```python
from build123d import *

# Parameters (mm, degrees)
DODANIE_WYCI_GNI_CIE1_DEPTH      = 85
SZKIC2_W                         = 10
SZKIC2_H                         = 10
WYTNIJ_WYCI_GNI_CIE1_DEPTH       = 80
DODANIE_WYCI_GNI_CIE3_DEPTH      = 80
DODANIE_WYCI_GNI_CIE3_DEPTH_BACK = 47
SZKIC4_W                         = 15.782842712
SZKIC4_H                         = 20
DODANIE_WYCI_GNI_CIE4_DEPTH      = 4
SZKIC5_W                         = 4
SZKIC5_H                         = 5
DODANIE_WYCI_GNI_CIE5_DEPTH      = 10
SZKIC6_W                         = 4
SZKIC6_H                         = 5
DODANIE_WYCI_GNI_CIE6_DEPTH      = 10
SFAZOWANIE1_SIZE                 = 1.5


with BuildPart() as part:
    # Szkic1 → Dodanie-wyci_gni_cie1 (new body)
    with BuildSketch(Plane.XY):
        Polygon((7.5, 0), (11.5, 4), (-10.578691808, 4), (-6.578691808, 0), align=None)
    extrude(amount=DODANIE_WYCI_GNI_CIE1_DEPTH)

    # Szkic2 → Wytnij-wyci_gni_cie1 (cut)
    with BuildSketch(Plane.XZ):
        with Locations((0.460654096, 21)):
            Rectangle(SZKIC2_W, SZKIC2_H)
        with Locations((0.460654096, 71)):
            Rectangle(SZKIC2_W, SZKIC2_H)
    extrude(amount=-WYTNIJ_WYCI_GNI_CIE1_DEPTH, mode=Mode.SUBTRACT)



with BuildPart() as body_2:
    # Szkic1_4 → Dodanie-wyci_gni_cie3 (new, two sides: drawn at the far end of the back side and taken through both)
    with BuildSketch(Plane.XY.offset(-DODANIE_WYCI_GNI_CIE3_DEPTH_BACK)):
        Polygon((19.282842712, 4), (23.282842712, 0), (26.717157288, 0), (30.717157288, 4), align=None)
    extrude(amount=DODANIE_WYCI_GNI_CIE3_DEPTH + DODANIE_WYCI_GNI_CIE3_DEPTH_BACK)


with BuildPart() as part_1:
    add(part.part)

    add(body_2.part)  # Dodanie-wyci_gni_cie4 merges body 2
    # Szkic4 → Dodanie-wyci_gni_cie4 (add)
    with BuildSketch(Plane.XZ):
        with Locations((15.391421356, 45)):
            Rectangle(SZKIC4_W, SZKIC4_H)
    extrude(amount=-DODANIE_WYCI_GNI_CIE4_DEPTH)

    # Szkic5 → Dodanie-wyci_gni_cie5 (add)
    with BuildSketch(Plane(origin=(0, 4, 0), x_dir=(1, 0, 0), z_dir=(0, 1, 0))):
        with Locations((25.460654096, -77.5)):
            Rectangle(SZKIC5_W, SZKIC5_H)
    extrude(amount=DODANIE_WYCI_GNI_CIE5_DEPTH)

    # Szkic6 → Dodanie-wyci_gni_cie6 (add)
    with BuildSketch(Plane(origin=(0, 4, 0), x_dir=(1, 0, 0), z_dir=(0, 1, 0))):
        with Locations((25.460654096, 44.5)):
            Rectangle(SZKIC6_W, SZKIC6_H)
    extrude(amount=DODANIE_WYCI_GNI_CIE6_DEPTH)

    # Sfazowanie1
    sfazowanie1_edges = [part_1.edges().sort_by_distance(p)[0] for p in [
        (0.460654096, 4, 76),
        (-4.539345904, 4, 71),
        (0.460654096, 4, 66),
        (5.460654096, 4, 71),
        (0.460654096, 4, 26),
        (-4.539345904, 4, 21),
        (0.460654096, 4, 16),
        (5.460654096, 4, 21),
    ]]
    chamfer(sfazowanie1_edges, length=SFAZOWANIE1_SIZE)


solid = part_1.part
```
Model file for the job. Use its own axes, mm. A direction names the side the tool comes from. Coordinates: 2 decimals unless noted, no trailing zeros. Order: outer loops, then holes, each group sorted by start corner. A loop starts at its lowest first (then second) coordinate and runs counter-clockwise, first axis right, second up. Notation, with made-up numbers: (58.25, 22.25) - (96.25, 22.25) arc R21 cw to (96.25, 48.25) - close; hole circle Ø7 at (-26, -19). An arc over 180 degrees is marked (long way). Return JSON: item names as keys, results as strings. Group by question number.
1) Saw through at C-C, the plane z = 71.5. Write the cut outline in (x, y), plus the area to 3 significant figures.
2) Saw through at D-D, the plane z = 53. Write the cut outline in (x, y), plus the area to 3 significant figures.
3) Probe line 1 (Y direction, x = -3.5, z = 45); line 2 (Z direction, x = 26, y = 4.75); line 3 (Z direction, x = 10.5, y = 2.25). List the from-to ranges inside material, lowest first. Write a range as from..to.
4) Saw through at A-A, the plane y = 10.75. Write the cut outline in (x, z).
5) Flat gauge pins, fed straight in: P1, Ø3, axis at x = 4, y = 2.5, coming from the -Z side; P2, Ø4, axis at x = 22, y = 3, coming from the +Z side; P3, Ø2.5, axis at y = 10.5, z = 78.5, coming from the +X side. Where does each tip first touch, or does it go through?
6) Saw through at B-B, the plane x = 4. Write the cut outline in (y, z), plus the area to 4 significant figures.
7) Mould opens along X. For faces 1 (the flat face through (0, 1, 16)), 2 (the flat face through (25, 14, 77)), 3 (the flat face through (5.461, 1, 71)), 4 (the flat face through (-8.61, 2.03, 41.9)) say: released by +X, released by -X, zero draft, split by the parting line, or undercut.
8) Tool access for faces 5 (the flat face through (25, 9, -42)), 6 (the flat face through (21.255, 2.028, 67.325)), 7 (the flat face through (9.5, 2, 17.3)), 8 (the flat face through (5.461, 1, 21)): list every direction of +Z, -Z, +X, -X, +Y, -Y with a clear straight run to the whole face (end or side of a thin tool).
Values found:
{
 "1": {"outline": "(-10.58, 4) - (-6.58, 0) - (-4.54, 0) - (-4.54, 2.5) - (-6.04, 4) - close; (5.46, 0) - (7.5, 0) - (11.5, 4) - (6.96, 4) - (5.46, 2.5) - close; (19.28, 4) - (23.28, 0) - (26.72, 0) - (30.72, 4) - close", "area": "59.8 mm²"},
 "2": {"outline": "(-10.58, 4) - (-6.58, 0) - (26.72, 0) - (30.72, 4) - close", "area": "149 mm²"},
 "3": {"line 1": "y = 0..4", "line 2": "z = -47..-42, 75..80", "line 3": "z = 35..55"},
 "4": {"outline": "(23.46, -47) - (27.46, -47) - (27.46, -42) - (23.46, -42) - close; (23.46, 75) - (27.46, 75) - (27.46, 80) - (23.46, 80) - close"},
 "5": {"P1": "stops at z = 0", "P2": "stops at z = 80", "P3": "stops at x = 27.46"},
 "6": {"outline": "(0, 0) - (4, 0) - (4, 14.5) - (2.5, 16) - (0, 16) - close; (0, 26) - (2.5, 26) - (4, 27.5) - (4, 64.5) - (2.5, 66) - (0, 66) - close; (0, 76) - (2.5, 76) - (4, 77.5) - (4, 85) - (0, 85) - close", "area": "255.5 mm²"},
 "7": {"face 1": "undercut", "face 2": "zero draft", "face 3": "undercut", "face 4": "released by -X"},
 "8": {"face 5": "+X, -X, +Y", "face 6": "+Z, -Y", "face 7": "-Z, -Y", "face 8": "+Y, -Y"}
}
